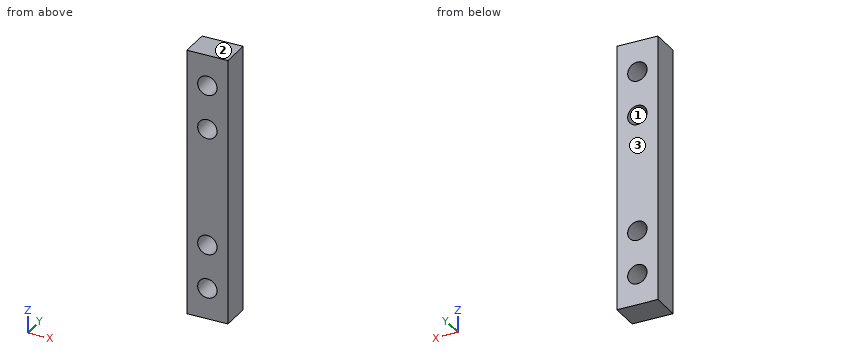
from build123d import *

# Parameters (mm, degrees)
SKETCH_1_W          = 7
SKETCH_1_H          = 45.5
EXTRUDE_1_DEPTH     = 5
CUT_EXTRUDE_1_REACH = 25.554
SKETCH_2_R          = 1.65
CUT_EXTRUDE_2_REACH = 25.554
SKETCH_3_R          = 1.65


with BuildPart() as part:
    # 草图1 → 凸台-拉伸1 (new body)
    with BuildSketch(Plane(origin=(0, 0, 0), x_dir=(1, 0, 0), z_dir=(0, 1, 0))):
        Rectangle(SKETCH_1_W, SKETCH_1_H)
    extrude(amount=EXTRUDE_1_DEPTH)

    # 草图2 → 切除-拉伸1 (cut, up to next)
    with BuildSketch(Plane(origin=(0, 5, 0), x_dir=(1, 0, 0), z_dir=(0, 1, 0)), mode=Mode.PRIVATE) as cut_extrude_1_sk1:
        with Locations(Location((0, 17.5, 0), (0, 0, 270))):
            Circle(SKETCH_2_R)
    cut_extrude_1_tool1 = extrude(cut_extrude_1_sk1.sketch, amount=-CUT_EXTRUDE_1_REACH, mode=Mode.PRIVATE) & part.part
    # 草图2 → 切除-拉伸1 (cut, up to next)
    with BuildSketch(Plane(origin=(0, 5, 0), x_dir=(1, 0, 0), z_dir=(0, 1, 0)), mode=Mode.PRIVATE) as cut_extrude_1_sk2:
        with Locations(Location((0, -17.5, 0), (0, 0, 270))):
            Circle(SKETCH_2_R)
    cut_extrude_1_tool2 = extrude(cut_extrude_1_sk2.sketch, amount=-CUT_EXTRUDE_1_REACH, mode=Mode.PRIVATE) & part.part
    add(cut_extrude_1_tool1.solids().sort_by_distance((0, 5, -17.5))[0], mode=Mode.SUBTRACT)
    add(cut_extrude_1_tool2.solids().sort_by_distance((0, 5, 17.5))[0], mode=Mode.SUBTRACT)

    # 草图3 → 切除-拉伸2 (cut, up to next)
    with BuildSketch(Plane(origin=(0, 5, 0), x_dir=(1, 0, 0), z_dir=(0, 1, 0)), mode=Mode.PRIVATE) as cut_extrude_2_sk1:
        with Locations(Location((0, 10, 0), (0, 0, 270))):
            Circle(SKETCH_3_R)
    cut_extrude_2_tool1 = extrude(cut_extrude_2_sk1.sketch, amount=-CUT_EXTRUDE_2_REACH, mode=Mode.PRIVATE) & part.part
    # 草图3 → 切除-拉伸2 (cut, up to next)
    with BuildSketch(Plane(origin=(0, 5, 0), x_dir=(1, 0, 0), z_dir=(0, 1, 0)), mode=Mode.PRIVATE) as cut_extrude_2_sk2:
        with Locations(Location((0, -10, 0), (0, 0, 270))):
            Circle(SKETCH_3_R)
    cut_extrude_2_tool2 = extrude(cut_extrude_2_sk2.sketch, amount=-CUT_EXTRUDE_2_REACH, mode=Mode.PRIVATE) & part.part
    add(cut_extrude_2_tool1.solids().sort_by_distance((0, 5, -10))[0], mode=Mode.SUBTRACT)
    add(cut_extrude_2_tool2.solids().sort_by_distance((0, 5, 10))[0], mode=Mode.SUBTRACT)


solid = part.part
Work out the finished part from the listing and answer in its coordinate system (mm). Face numbers are marked on the shaded views. Coordinates: 2 decimals unless noted, no trailing zeros. Write each loop counter-clockwise with the first axis right and the second up, starting at its lowest first coordinate (ties: lowest second). Pieces come first, ordered by that corner, then holes. Notation, with made-up numbers: (68, 46) - (95, 46) arc R26 ccw to (95, 71) - close; hole circle Ø4 at (-39.5, 7.5). An arc over 180 degrees is marked (long way). One line per question, with ' | ' between items.
1) Find section A-A, the plane z = -10. Determine the outline of the cut face in (x, y).
Checks:
outline: (-3.5, 0) - (-1.65, 0) - (-1.65, 5) - (-3.5, 5) - close; (1.65, 0) - (3.5, 0) - (3.5, 5) - (1.65, 5) - close
2) Find section B-B, the plane x = 0. Determine the outline of the cut face in (y, z), and give its area (4 significant figures).
Checks:
outline: (0, -22.75) - (5, -22.75) - (5, -19.15) - (0, -19.15) - close; (0, -15.85) - (5, -15.85) - (5, -11.65) - (0, -11.65) - close; (0, -8.35) - (5, -8.35) - (5, 8.35) - (0, 8.35) - close; (0, 11.65) - (5, 11.65) - (5, 15.85) - (0, 15.85) - close; (0, 19.15) - (5, 19.15) - (5, 22.75) - (0, 22.75) - close | area: 161.5 mm2
3) Find section C-C, the plane y = 1.7. Determine the outline of the cut face in (x, z), and give its area (3 significant figures).
Checks:
outline: (-3.5, -22.75) - (3.5, -22.75) - (3.5, 22.75) - (-3.5, 22.75) - close; hole circle Ø3.3 at (0, -17.5); hole circle Ø3.3 at (0, -10); hole circle Ø3.3 at (0, 10); hole circle Ø3.3 at (0, 17.5) | area: 284 mm2
4) Consider probe 1 along Z at (x, y) = (-0.75, 1.05); probe 2 along X at (y, z) = (1.3, 17.5); probe 3 along X at (y, z) = (0.6, 11). Determine where each line is inside the solid, lowest interval first. Write a range as [from, to].
Checks:
probe 1: [-22.75, -18.97], [-16.03, -11.47], [-8.53, 8.53], [11.47, 16.03], [18.97, 22.75] | probe 2: [-3.5, -1.65], [1.65, 3.5] | probe 3: [-3.5, -1.31], [1.31, 3.5]
5) The mould has two halves that part along Z. Classify the marked faces 1, 2 and 3: +Z half, -Z half, draft (parallel to the pull), parting line (faces both ways), or undercut.
Checks:
face 1: undercut | face 2: +Z half | face 3: draft
6) Find section D-D, the plane z = -17. Determine the outline of the cut face in (x, y).
Checks:
outline: (-3.5, 0) - (-1.57, 0) - (-1.57, 5) - (-3.5, 5) - close; (1.57, 0) - (3.5, 0) - (3.5, 5) - (1.57, 5) - close
